```python
from build123d import *

# Parameters (mm, degrees)
F0_R     = 7.95
F1_DEPTH = 3.7
F2_R     = 8.75
F3_DEPTH = 3.5
F4_R     = 7.95
F5_DEPTH = 3.7
F6_R     = 2.0190036786
F7_DEPTH = 10.901


with BuildPart() as f1:
    # F0 (on Top) → F1 (new body)
    with BuildSketch(Plane.XY):
        Circle(F0_R)
    extrude(amount=F1_DEPTH)

    # F2 (on face) → F3 (join)
    with BuildSketch(Plane.XY.offset(3.7)):
        Circle(F2_R)
    extrude(amount=F3_DEPTH)

    # F4 (on face) → F5 (join)
    with BuildSketch(Plane.XY.offset(7.2)):
        Circle(F4_R)
    extrude(amount=F5_DEPTH)

    # F6 (on face) → F7 (cut, through all)
    with BuildSketch(Plane.XY.offset(10.9)):
        with Locations((-5.1206611768, 0)):
            Circle(F6_R)
        with Locations((2.5603305884, -4.4346226633)):
            Circle(F6_R)
        with Locations((2.5603305884, 4.4346226633)):
            Circle(F6_R)
    extrude(amount=-F7_DEPTH, mode=Mode.SUBTRACT)


solid = f1.part
```
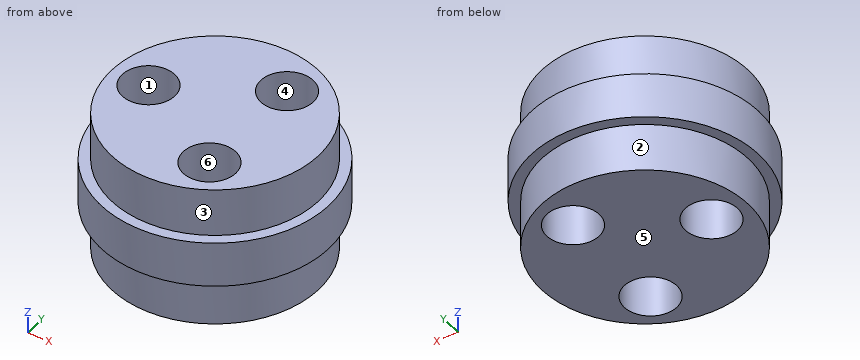
Design review of the part built by this model. Coordinates are the model's own, in mm. Face numbers are marked on the shaded views. A direction names the side the tool comes from. Coordinates: 2 decimals unless noted, no trailing zeros. Loops run counter-clockwise (first coordinate to the right, second up) from the corner with the lowest first, then second, coordinate; pieces in that order, holes last. Notation, with made-up numbers: (-33, -22.75) - (-17, -22.75) arc R32 cw to (-17, 9.25) - close; hole circle Ø6 at (15.5, 66.25). An arc over 180 degrees is marked (long way). Use CSV: the item, a comma, the result in double quotes. Start each with the question number.
1) Consider section A-A on y = 0. Write out the cut boundary in (x, z).
2) The part is to be moulded in two halves that separate along X. For the marked faces 3, 4, 5 and 6, say which applies: +X half, -X half, draft (parallel to the pull), parting line (faces both ways), or undercut.
3) Consider section B-B on x = 0. Write out the cut boundary in (y, z), then the cut area to 3 significant figures.
4) Consider section D-D on x = 3. Write out the cut boundary in (y, z), then the cut area to 3 significant figures.
5) For pin 1 Ø3 at (x, y) = (-5.12, 0) entering from +Z; pin 2 Ø1 at (x, z) = (-2, 3.5) entering from -Y; pin 3 Ø4 at (y, z) = (-6, 7) entering from -X; pin 4 Ø2 at (y, z) = (2.5, 6.5) entering from -X, all flat-tipped, find the tip position at first contact; note any pin that passes through.
6) Wall thickness on L1, parallel to Y at x = 1.5, z = 5.25; L2, parallel to X at y = 0.75, z = 3.75; L3, parallel to Y at x = -6, z = 8.5: over which ranges is each line inside the solid? List them lowest first. Write a range as from..to.
7) Consider section C-C on x = -5.75. Write out the cut boundary in (y, z).
8) Tool access review of the marked faces 1 and 2: name each direction out of +Z, -Z, +X, -X, +Y, -Y from which nothing blocks a thin tool from reaching the whole face with its end or side.
Geometry says:
1,outline,"(-8.75, 3.7) - (-7.95, 3.7) - (-7.95, 0) - (-7.14, 0) - (-7.14, 10.9) - (-7.95, 10.9) - (-7.95, 7.2) - (-8.75, 7.2) - close; (-3.1, 0) - (7.95, 0) - (7.95, 3.7) - (8.75, 3.7) - (8.75, 7.2) - (7.95, 7.2) - (7.95, 10.9) - (-3.1, 10.9) - close"
2,face 3,"parting line"
2,face 4,"undercut"
2,face 5,"draft"
2,face 6,"undercut"
3,outline,"(-8.75, 3.7) - (-7.95, 3.7) - (-7.95, 0) - (7.95, 0) - (7.95, 3.7) - (8.75, 3.7) - (8.75, 7.2) - (7.95, 7.2) - (7.95, 10.9) - (-7.95, 10.9) - (-7.95, 7.2) - (-8.75, 7.2) - close"
3,area,"179 mm^2"
4,outline,"(-8.22, 3.7) - (-7.36, 3.7) - (-7.36, 0) - (-6.41, 0) - (-6.41, 10.9) - (-7.36, 10.9) - (-7.36, 7.2) - (-8.22, 7.2) - close; (-2.46, 0) - (2.46, 0) - (2.46, 10.9) - (-2.46, 10.9) - close; (6.41, 0) - (7.36, 0) - (7.36, 3.7) - (8.22, 3.7) - (8.22, 7.2) - (7.36, 7.2) - (7.36, 10.9) - (6.41, 10.9) - close"
4,area,"80.6 mm^2"
5,pin 1,"through"
5,pin 2,"y = -8.61"
5,pin 3,"x = -7.78"
5,pin 4,"x = -8.62"
6,L1,"-8.62..-6.15, -2.72..2.72, 6.15..8.62"
6,L2,"-8.72..-7, -3.25..8.72"
6,L3,"-5.22..-1.82, 1.82..5.22"
7,outline,"(-6.6, 3.7) - (-5.49, 3.7) - (-5.49, 0) - (-1.92, 0) - (-1.92, 10.9) - (-5.49, 10.9) - (-5.49, 7.2) - (-6.6, 7.2) - close; (1.92, 0) - (5.49, 0) - (5.49, 3.7) - (6.6, 3.7) - (6.6, 7.2) - (5.49, 7.2) - (5.49, 10.9) - (1.92, 10.9) - close"
8,face 1,"+Z, -Z"
8,face 2,"-Z"
